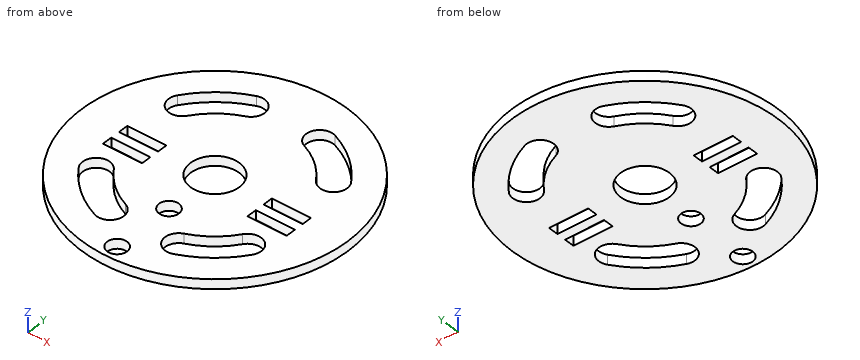
from build123d import *

# Parameters (mm, degrees)
SKETCH_1_R      = 27.5
SKETCH_1_R_2    = 5.05
SKETCH_1_R_3    = 2.05
SKETCH_1_W      = 8.1
SKETCH_1_H      = 2.1
EXTRUDE_1_DEPTH = 2


with BuildPart() as part:
    # 草图1 → 凸台-拉伸1 (new body)
    with BuildSketch(Plane.XY):
        with Locations((0, 4)):
            Circle(SKETCH_1_R)
        with Locations((0, 4)):
            Circle(SKETCH_1_R_2, mode=Mode.SUBTRACT)
        with Locations((0, -7.5)):
            Circle(SKETCH_1_R_3, mode=Mode.SUBTRACT)
        with Locations((0, -20.5)):
            Circle(SKETCH_1_R_3, mode=Mode.SUBTRACT)
        with Locations((-15, 4)):
            Rectangle(SKETCH_1_W, SKETCH_1_H, mode=Mode.SUBTRACT)
        with Locations((-15, 0)):
            Rectangle(SKETCH_1_W, SKETCH_1_H, mode=Mode.SUBTRACT)
        with Locations((15, 4)):
            Rectangle(SKETCH_1_W, SKETCH_1_H, mode=Mode.SUBTRACT)
        with Locations((15, 0)):
            Rectangle(SKETCH_1_W, SKETCH_1_H, mode=Mode.SUBTRACT)
        with BuildLine():
            ThreePointArc((-18.02272766, -8.370387974), (-13.679746228, -13.050212729), (-8.169823727, -16.275581156))
            ThreePointArc((-8.169823727, -16.275581156), (-4.506388665, -14.716501354), (-6.065468468, -11.053066292))
            ThreePointArc((-6.065468468, -11.053066292), (-10.156163971, -8.658477236), (-13.380495097, -5.184065739))
            ThreePointArc((-13.380495097, -5.184065739), (-17.294772496, -4.456110575), (-18.02272766, -8.370387974))
        make_face(mode=Mode.SUBTRACT)
        with BuildLine():
            ThreePointArc((18.02272766, -8.370387974), (13.679746228, -13.050212729), (8.169823727, -16.275581156))
            ThreePointArc((8.169823727, -16.275581156), (4.506388665, -14.716501354), (6.065468468, -11.053066292))
            ThreePointArc((6.065468468, -11.053066292), (10.156163971, -8.658477236), (13.380495097, -5.184065739))
            ThreePointArc((13.380495097, -5.184065739), (17.294772496, -4.456110575), (18.02272766, -8.370387974))
        make_face(mode=Mode.SUBTRACT)
        with BuildLine():
            ThreePointArc((18.02272766, 16.370387974), (13.679746228, 21.050212729), (8.169823727, 24.275581156))
            ThreePointArc((8.169823727, 24.275581156), (4.506388665, 22.716501354), (6.065468468, 19.053066292))
            ThreePointArc((6.065468468, 19.053066292), (10.156163971, 16.658477236), (13.380495097, 13.184065739))
            ThreePointArc((13.380495097, 13.184065739), (17.294772496, 12.456110575), (18.02272766, 16.370387974))
        make_face(mode=Mode.SUBTRACT)
        with BuildLine():
            ThreePointArc((-18.02272766, 16.370387974), (-13.679746228, 21.050212729), (-8.169823727, 24.275581156))
            ThreePointArc((-8.169823727, 24.275581156), (-4.506388665, 22.716501354), (-6.065468468, 19.053066292))
            ThreePointArc((-6.065468468, 19.053066292), (-10.156163971, 16.658477236), (-13.380495097, 13.184065739))
            ThreePointArc((-13.380495097, 13.184065739), (-17.294772496, 12.456110575), (-18.02272766, 16.370387974))
        make_face(mode=Mode.SUBTRACT)
    extrude(amount=EXTRUDE_1_DEPTH)


solid = part.part
Design review of the part built by this model. Coordinates are the model's own, in mm. Round coordinates to 2 decimals unless told otherwise and drop trailing zeros. Write each loop counter-clockwise with the first axis right and the second up, starting at its lowest first coordinate (ties: lowest second). Pieces come first, ordered by that corner, then holes. Notation, with made-up numbers: (75, 79.25) - (82, 79.25) arc R10 ccw to (82, 91.25) - close; hole circle Ø10 at (35.5, 55.5). An arc over 180 degrees is marked (long way). Return JSON: item names as keys, results as strings. Group by question number.
Item 1: For probe 1 along Y at (x, z) = (0, 0.9); probe 2 along X at (y, z) = (3.5, 1.15); probe 3 along Y at (x, z) = (-18, 1), list the stretches that pass through material, from the lowest coordinate up. Write a range as [from, to].
Item 2: We need section D-D on z = 0.65. Give the number of separate pieces and of enclosed holes in the cut face, and give its area (3 significant figures).
Item 3: We need section A-A on y = -20.5. Write out the cut boundary in (x, z), and give its area (3 significant figures).
Item 4: We need section C-C on y = -7.5. Write out the cut boundary in (x, z), and give its area (3 significant figures).
Item 5: We need section B-B on x = 0. Write out the cut boundary in (y, z).
Item 6: Insertion check: P1, Ø1, axis at y = -0.5, z = 1, coming from the +X side; P2, Ø1, axis at y = 0, z = 1.5, coming from the +X side; P3, Ø0.6, axis at y = 0, z = 1.5, coming from the -X side. Each pin has a flat end and moves straight along its axis. Give the tip position at first contact, or say it passes through.
Model answer:
{
 "1": {"probe 1": "y = [-23.5, -22.55], [-18.45, -9.55], [-5.45, -1.05], [9.05, 31.5]", "probe 2": "x = [-27.5, -19.05], [-10.95, -5.03], [5.03, 10.95], [19.05, 27.5]", "probe 3": "y = [-16.79, -8.4], [-5.15, -1.05], [1.05, 2.95], [5.05, 13.15], [16.4, 24.79]"},
 "2": {"separate pieces": "1", "enclosed holes": "11", "area": "1,850 mm²"},
 "3": {"outline": "(-12.49, 0) - (-2.05, 0) - (-2.05, 2) - (-12.49, 2) - close; (2.05, 0) - (12.49, 0) - (12.49, 2) - (2.05, 2) - close", "area": "41.8 mm²"},
 "4": {"outline": "(-24.98, 0) - (-18.42, 0) - (-18.42, 2) - (-24.98, 2) - close; (-11.45, 0) - (-2.05, 0) - (-2.05, 2) - (-11.45, 2) - close; (2.05, 0) - (11.45, 0) - (11.45, 2) - (2.05, 2) - close; (18.42, 0) - (24.98, 0) - (24.98, 2) - (18.42, 2) - close", "area": "63.8 mm²"},
 "5": {"outline": "(-23.5, 0) - (-22.55, 0) - (-22.55, 2) - (-23.5, 2) - close; (-18.45, 0) - (-9.55, 0) - (-9.55, 2) - (-18.45, 2) - close; (-5.45, 0) - (-1.05, 0) - (-1.05, 2) - (-5.45, 2) - close; (9.05, 0) - (31.5, 0) - (31.5, 2) - (9.05, 2) - close"},
 "6": {"P1": "stops at x = 27.21", "P2": "stops at x = 27.28", "P3": "stops at x = -27.25"}
}
